```python
from build123d import *

# Parameters (mm, degrees)
SKETCH1_R           = 1.5
BOSS_EXTRUDE1_DEPTH = 5


with BuildPart() as part:
    # Sketch1 → Boss-Extrude1 (new body)
    with BuildSketch(Plane.XY):
        with BuildLine():
            Line((-91.35, 42.09), (-91.35, -42.09))
            Line((-91.35, -42.09), (91.35, -42.09))
            Line((91.35, -42.09), (91.35, -9.373756295))
            Line((91.35, -9.373756295), (8.343053199, -9.373756295))
            ThreePointArc((8.343053199, -9.373756295), (5.843053199, -6.873756295), (8.343053199, -4.373756295))
            Line((8.343053199, -4.373756295), (91.35, -4.373756295))
            Line((91.35, -4.373756295), (91.35, 42.09))
            Line((91.35, 42.09), (-91.35, 42.09))
        make_face()
        with BuildLine():
            ThreePointArc((-40.489979298, -20.16630551), (-48.867123378, -25.905481248), (-58.308825968, -29.642984865))
            ThreePointArc((-58.308825968, -29.642984865), (-60.149390448, -28.588317906), (-59.094723489, -26.747753426))
            ThreePointArc((-59.094723489, -26.747753426), (-50.275796541, -23.25677592), (-42.451209718, -17.896156784))
            ThreePointArc((-42.451209718, -17.896156784), (-40.846464239, -17.667243828), (-39.970594508, -19.031231147))
            ThreePointArc((-39.970594508, -19.031231147), (-40.106607189, -19.655361416), (-40.489979298, -20.16630551))
        make_face(mode=Mode.SUBTRACT)
        with BuildLine():
            ThreePointArc((-65.144358521, -17.951194504), (-76.122435192, -17.811173415), (-86.43146485, -14.034709351))
            ThreePointArc((-86.43146485, -14.034709351), (-86.987178316, -11.987471568), (-84.939940533, -11.431758101))
            ThreePointArc((-84.939940533, -11.431758101), (-78.516125038, -14.163976019), (-71.631092615, -15.315821832))
            ThreePointArc((-71.631092615, -15.315821832), (-75.191833702, -4.546421602), (-67.344295246, 3.643511155))
            ThreePointArc((-67.344295246, 3.643511155), (-65.062648548, 4.546702365), (-63.038259097, 5.933610208))
            ThreePointArc((-63.038259097, 5.933610208), (-51.860585441, 7.861943698), (-44.921737847, -1.110862578))
            ThreePointArc((-44.921737847, -1.110862578), (-42.027839791, 5.241756905), (-40.702136642, 12.095437041))
            ThreePointArc((-40.702136642, 12.095437041), (-39.151472366, 13.485222207), (-37.706118198, 11.986217927))
            ThreePointArc((-37.706118198, 11.986217927), (-37.707113918, 11.931572095), (-37.710099754, 11.876998812))
            ThreePointArc((-37.710099754, 11.876998812), (-40.341925186, 1.21814014), (-46.362913364, -7.96257196))
            ThreePointArc((-46.362913364, -7.96257196), (-47.396661948, -9.432315012), (-48.655902683, -10.714147119))
            ThreePointArc((-48.655902683, -10.714147119), (-54.732378683, -14.877136713), (-61.581046755, -17.588186064))
            ThreePointArc((-61.581046755, -17.588186064), (-63.34782833, -17.915697351), (-65.144358521, -17.951194504))
        make_face(mode=Mode.SUBTRACT)
        with Locations((-70.223567272, 14.250694236)):
            Circle(SKETCH1_R, mode=Mode.SUBTRACT)
    extrude(amount=BOSS_EXTRUDE1_DEPTH)


solid = part.part
```
Here's how the part is built. I have some questions about the finished solid (model axes, mm). A direction names the side the tool comes from. Give positions to 0.01 mm unless a question says otherwise; leave off trailing zeros. Loops run counter-clockwise (first coordinate to the right, second up) from the corner with the lowest first, then second, coordinate; pieces in that order, holes last. Notation, with made-up numbers: (-23, 59.25) -> (-9, 59.25) arc R10 cw to (-9, 65.25) -> close; hole circle Ø7 at (86.5, 37). An arc over 180 degrees is marked (long way). Use one line per item in the form item = value. Start each with the question number.
1) Imagine slicing it at B-B (z = 3.45). Please give me the cut outline in (x, y).
2) For P1, Ø2.5, axis at x = -70.22, y = 14.25, coming from the -Z side, with a flat end and sliding along its axis, tell me the tip position at first contact or that it passes through.
3) Thinking about a two-plate mould opening in X: for faces 4 (the face through (-1, -42.09, 2)), 5 (the face through (-75.97, -17.84, 2.46)), 6 (the face through (-63.323, -17.913, 2.465)), 7 (the face through (91.35, 19, 2)), which applies, +X half, -X half, draft (parallel to the pull), parting line (faces both ways), or undercut?
4) Please list where these lines run through material, in increasing order: line 1 along Y through (x, z) = (71, 0.45); line 2 along Y through (x, z) = (-53, 2.8); line 3 along X through (y, z) = (-11.5, 0.75).
5) Which directions (+Z, -Z, +X, -X, +Y, -Y) give clear straight access to the entire face, cutting with the end or side of a thin tool? Please do faces 1 (the face through (1, 42.09, 2)), 2 (the face through (-52.017, 7.921, 2.465)), 3 (the face through (50, -9.374, 2)).
6) Imagine slicing it at A-A (x = 42.5). Please give me the cut outline in (y, z).
Check values:
q1.outline = (-91.35, -42.09) -> (91.35, -42.09) -> (91.35, -9.37) -> (8.34, -9.37) arc R2.5 cw to (8.34, -4.37) -> (91.35, -4.37) -> (91.35, 42.09) -> (-91.35, 42.09) -> close; hole (-86.43, -14.03) arc R32.6 ccw to (-65.14, -17.95) arc R11 ccw to (-61.58, -17.59) arc R32.99 ccw to (-48.66, -10.71) arc R11 ccw to (-46.36, -7.96) arc R32.6 ccw to (-37.71, 11.88) arc R1.5 ccw to (-40.7, 12.1) arc R29.6 cw to (-44.92, -1.11) arc R11 ccw to (-63.04, 5.93) arc R10.99 cw to (-67.34, 3.64) arc R11 ccw to (-71.63, -15.32) arc R29.6 cw to (-84.94, -11.43) arc R1.5 ccw to start; hole circle Ø3 at (-70.22, 14.25); hole (-59.09, -26.75) arc R1.5 ccw to (-58.31, -29.64) arc R45.48 ccw to (-40.49, -20.17) arc R1.5 ccw to (-42.45, -17.9) arc R42.48 cw to start
q2.P1 = through
q3.face_4 = draft
q3.face_5 = undercut
q3.face_6 = undercut
q3.face_7 = +X half
q4.line_1 = -42.09 to -9.37, -4.37 to 42.09
q4.line_2 = -42.09 to -27.84, -24.58 to -13.89, 8.23 to 42.09
q4.line_3 = -91.35 to -86.54, -84.82 to -74.49, -49.6 to 91.35
q5.face_1 = +Z, -Z, +X, -X, +Y
q5.face_2 = +Z, -Z
q5.face_3 = +Z, -Z, +X
q6.outline = (-42.09, 0) -> (-9.37, 0) -> (-9.37, 5) -> (-42.09, 5) -> close; (-4.37, 0) -> (42.09, 0) -> (42.09, 5) -> (-4.37, 5) -> close
